```python
from build123d import *

# Parameters (mm, degrees)
F0_W     = 80
F0_H     = 300
F0_R     = 10
F1_DEPTH = 10
F2_SIZE2 = 5
F2_SIZE  = 5


with BuildPart() as f1:
    # F0 (on Top) → F1 (new body)
    with BuildSketch(Plane.XY):
        Rectangle(F0_W, F0_H)
        with Locations((0, -110)):
            Circle(F0_R, mode=Mode.SUBTRACT)
        with Locations((0, 110)):
            Circle(F0_R, mode=Mode.SUBTRACT)
    extrude(amount=-F1_DEPTH)

    # F2
    f2_edges = [f1.edges().sort_by_distance(p)[0] for p in [
        (40, 150, -5),
        (40, -150, -5),
        (-40, -150, -5),
        (-40, 150, -5),
    ]]
    chamfer(f2_edges, length=F2_SIZE, length2=F2_SIZE2)


solid = f1.part
```
Here's how the part is built. I have some questions about the finished solid (model axes, mm). Coordinates: 2 decimals unless noted, no trailing zeros. Order: outer loops, then holes, each group sorted by start corner. A loop starts at its lowest first (then second) coordinate and runs counter-clockwise, first axis right, second up. Notation, with made-up numbers: (86, 89) - (110, 89) arc R10 ccw to (110, 107) - close; hole circle Ø7 at (-2.75, 42). An arc over 180 degrees is marked (long way). One line per question, with ' | ' between items.
(1) Suppose I cut it at B-B on x = 0. List the corners of the cut face in (y, z) for me.
Report:
outline: (-150, -10) - (-120, -10) - (-120, 0) - (-150, 0) - close; (-100, -10) - (100, -10) - (100, 0) - (-100, 0) - close; (120, -10) - (150, -10) - (150, 0) - (120, 0) - close
(2) If we mould it in two halves opening along Y, with no side actions, what happens to faces 1 (the flat face through (-37, -148, -5)), 2 (the flat face through (-40, -2, -5)), 3 (the cylindrical face through (-1.302, -100.085, -4.93))? For each: pulls with the +Y half, pulls with the -Y half, needs draft (parallel to the pull), parting line crosses it, or undercut.
Report:
face 1: pulls with the -Y half | face 2: needs draft | face 3: undercut
(3) Suppose I cut it at A-A on y = -110. List the corners of the cut face in (x, z) for me.
Report:
outline: (-40, -10) - (-10, -10) - (-10, 0) - (-40, 0) - close; (10, -10) - (40, -10) - (40, 0) - (10, 0) - close
(4) If I drill on L1, parallel to Y at x = 0, z = -5.5; L2, parallel to Y at x = 2, z = -4.5; L3, parallel to X at y = -104, z = -5, over which ranges is the centre line in solid material (lowest first)?
Report:
L1: y = -150 to -120, -100 to 100, 120 to 150 | L2: y = -150 to -119.8, -100.2 to 100.2, 119.8 to 150 | L3: x = -40 to -8, 8 to 40
(5) Suppose I cut it at C-C on z = -3.5. List the corners of the cut face in (x, y) for me.
Report:
outline: (-40, -145) - (-35, -150) - (35, -150) - (40, -145) - (40, 145) - (35, 150) - (-35, 150) - (-40, 145) - close; hole circle Ø20 at (0, -110); hole circle Ø20 at (0, 110)
